from build123d import *

# Parameters (mm, degrees)
PLACA_DELANTERA_START               = -206
PLACA_DELANTERA_DEPTH               = 3
AGUJERO_PLACA_DELANTERA_1_PROFILE_R = 2
AGUJERO_PLACA_DELANTERA_2_PROFILE_R = 2
AGUJERO_PLACA_DELANTERA_3_PROFILE_R = 2
AGUJERO_PLACA_DELANTERA_4_PROFILE_R = 2
PLACA_TRASERA_START                 = -142
PLACA_TRASERA_DEPTH                 = 3
AGUJERO_PLACA_TRASERA_1_PROFILE_R   = 2
AGUJERO_PLACA_TRASERA_2_PROFILE_R   = 2
AGUJERO_PLACA_TRASERA_3_PROFILE_R   = 2
AGUJERO_PLACA_TRASERA_4_PROFILE_R   = 2
MARCO_INTERIOR_START                = -86
SK_MARCO_INTERIOR_W                 = 64
SK_MARCO_INTERIOR_H                 = 26
SK_MARCO_INTERIOR_R                 = 11
MARCO_INTERIOR_DEPTH                = 3
MARCO_EXTERIOR_START                = -143
SK_MARCO_EXTERIOR_W                 = 64
SK_MARCO_EXTERIOR_H                 = 26
SK_MARCO_EXTERIOR_R                 = 11
MARCO_EXTERIOR_DEPTH                = 3
CORTAR_EXTRUIR2_DEPTH               = 10


with BuildPart() as part:
    # Sk_Eje_cuerpo → Eje_cuerpo (revolve)
    with BuildSketch(Plane(origin=(0, 0, 0), x_dir=(1, 0, 0), z_dir=(0, 1, 0)), mode=Mode.PRIVATE) as eje_cuerpo_sk:
        Polygon((-183.5, 84), (-186, 84), (-186, 92), (-182.5, 92), (-182.5, 138), (-186, 138), (-186, 146), (-185.3, 149), (-183.3, 152), (-180, 154.5), (-176.5, 155.7), (-172.5, 156), (-172.5, 147), (-183.5, 147), (-183.5, 138.5), (-178.8, 138.5), (-178.8, 91.5), (-183.5, 91.5), align=None)
    revolve(eje_cuerpo_sk.sketch.rotate(Axis((-172.5, 0, -62.1), (0, 0, -1)), 180), axis=Axis((-172.5, 0, -62.1), (0, 0, -1)))



with BuildPart() as body_2:
    # Sk_Placa_delantera → Placa_delantera (new body)
    with BuildSketch(Plane(origin=(0, 0, 0), x_dir=(0, 0, -1), z_dir=(1, 0, 0)).offset(PLACA_DELANTERA_START)):
        Polygon((86, -12), (112, -12), (116, -22), (120, -12), (146, -12), (146, 10), (144.125, 14), (142.25, 10), (140.375, 14), (138.5, 10), (136.625, 14), (134.75, 10), (132.875, 14), (131, 10), (129.125, 14), (127.25, 10), (125.375, 14), (123.5, 10), (121.625, 14), (119.75, 10), (117.875, 14), (116, 10), (114.125, 14), (112.25, 10), (110.375, 14), (108.5, 10), (106.625, 14), (104.75, 10), (102.875, 14), (101, 10), (99.125, 14), (97.25, 10), (95.375, 14), (93.5, 10), (91.625, 14), (89.75, 10), (87.875, 14), (86, 10), align=None)
    extrude(amount=PLACA_DELANTERA_DEPTH)

    # Agujero_Placa_delantera_1: sweep along a curve in space
    with BuildLine() as agujero_placa_delantera_1_path:
        Line((-201.5, -6, -91), (-207.5, -6, -91))
    # Agujero_Placa_delantera_1 profile (on start of the path) → Agujero_Placa_delantera_1 (sweep, cut)
    with BuildSketch(Plane(origin=(-201.5, -6, -91), x_dir=(0, 0, -1), z_dir=(-1, 0, 0))):
        Circle(AGUJERO_PLACA_DELANTERA_1_PROFILE_R)
    sweep(path=agujero_placa_delantera_1_path.line, mode=Mode.SUBTRACT)

    # Agujero_Placa_delantera_2: sweep along a curve in space
    with BuildLine() as agujero_placa_delantera_2_path:
        Line((-201.5, 2, -91), (-207.5, 2, -91))
    # Agujero_Placa_delantera_2 profile (on start of the path) → Agujero_Placa_delantera_2 (sweep, cut)
    with BuildSketch(Plane(origin=(-201.5, 2, -91), x_dir=(0, 0, -1), z_dir=(-1, 0, 0))):
        Circle(AGUJERO_PLACA_DELANTERA_2_PROFILE_R)
    sweep(path=agujero_placa_delantera_2_path.line, mode=Mode.SUBTRACT)

    # Agujero_Placa_delantera_3: sweep along a curve in space
    with BuildLine() as agujero_placa_delantera_3_path:
        Line((-201.5, -6, -141), (-207.5, -6, -141))
    # Agujero_Placa_delantera_3 profile (on start of the path) → Agujero_Placa_delantera_3 (sweep, cut)
    with BuildSketch(Plane(origin=(-201.5, -6, -141), x_dir=(0, 0, -1), z_dir=(-1, 0, 0))):
        Circle(AGUJERO_PLACA_DELANTERA_3_PROFILE_R)
    sweep(path=agujero_placa_delantera_3_path.line, mode=Mode.SUBTRACT)

    # Agujero_Placa_delantera_4: sweep along a curve in space
    with BuildLine() as agujero_placa_delantera_4_path:
        Line((-201.5, 2, -141), (-207.5, 2, -141))
    # Agujero_Placa_delantera_4 profile (on start of the path) → Agujero_Placa_delantera_4 (sweep, cut)
    with BuildSketch(Plane(origin=(-201.5, 2, -141), x_dir=(0, 0, -1), z_dir=(-1, 0, 0))):
        Circle(AGUJERO_PLACA_DELANTERA_4_PROFILE_R)
    sweep(path=agujero_placa_delantera_4_path.line, mode=Mode.SUBTRACT)


with BuildPart() as body_3:
    # Sk_Placa_trasera → Placa_trasera (new body)
    with BuildSketch(Plane(origin=(0, 0, 0), x_dir=(0, 0, -1), z_dir=(1, 0, 0)).offset(PLACA_TRASERA_START)):
        Polygon((86, -12), (146, -12), (146, 10), (144.125, 14), (142.25, 10), (140.375, 14), (138.5, 10), (136.625, 14), (134.75, 10), (132.875, 14), (131, 10), (129.125, 14), (127.25, 10), (125.375, 14), (123.5, 10), (121.625, 14), (119.75, 10), (117.875, 14), (116, 10), (114.125, 14), (112.25, 10), (110.375, 14), (108.5, 10), (106.625, 14), (104.75, 10), (102.875, 14), (101, 10), (99.125, 14), (97.25, 10), (95.375, 14), (93.5, 10), (91.625, 14), (89.75, 10), (87.875, 14), (86, 10), align=None)
    extrude(amount=PLACA_TRASERA_DEPTH)

    # Agujero_Placa_trasera_1: sweep along a curve in space
    with BuildLine() as agujero_placa_trasera_1_path:
        Line((-137.5, -6, -91), (-143.5, -6, -91))
    # Agujero_Placa_trasera_1 profile (on start of the path) → Agujero_Placa_trasera_1 (sweep, cut)
    with BuildSketch(Plane(origin=(-137.5, -6, -91), x_dir=(0, 0, -1), z_dir=(-1, 0, 0))):
        Circle(AGUJERO_PLACA_TRASERA_1_PROFILE_R)
    sweep(path=agujero_placa_trasera_1_path.line, mode=Mode.SUBTRACT)

    # Agujero_Placa_trasera_2: sweep along a curve in space
    with BuildLine() as agujero_placa_trasera_2_path:
        Line((-137.5, 2, -91), (-143.5, 2, -91))
    # Agujero_Placa_trasera_2 profile (on start of the path) → Agujero_Placa_trasera_2 (sweep, cut)
    with BuildSketch(Plane(origin=(-137.5, 2, -91), x_dir=(0, 0, -1), z_dir=(-1, 0, 0))):
        Circle(AGUJERO_PLACA_TRASERA_2_PROFILE_R)
    sweep(path=agujero_placa_trasera_2_path.line, mode=Mode.SUBTRACT)

    # Agujero_Placa_trasera_3: sweep along a curve in space
    with BuildLine() as agujero_placa_trasera_3_path:
        Line((-137.5, -6, -141), (-143.5, -6, -141))
    # Agujero_Placa_trasera_3 profile (on start of the path) → Agujero_Placa_trasera_3 (sweep, cut)
    with BuildSketch(Plane(origin=(-137.5, -6, -141), x_dir=(0, 0, -1), z_dir=(-1, 0, 0))):
        Circle(AGUJERO_PLACA_TRASERA_3_PROFILE_R)
    sweep(path=agujero_placa_trasera_3_path.line, mode=Mode.SUBTRACT)

    # Agujero_Placa_trasera_4: sweep along a curve in space
    with BuildLine() as agujero_placa_trasera_4_path:
        Line((-137.5, 2, -141), (-143.5, 2, -141))
    # Agujero_Placa_trasera_4 profile (on start of the path) → Agujero_Placa_trasera_4 (sweep, cut)
    with BuildSketch(Plane(origin=(-137.5, 2, -141), x_dir=(0, 0, -1), z_dir=(-1, 0, 0))):
        Circle(AGUJERO_PLACA_TRASERA_4_PROFILE_R)
    sweep(path=agujero_placa_trasera_4_path.line, mode=Mode.SUBTRACT)


with BuildPart() as part_1:
    add(part.part)

    add(body_2.part)  # Marco_interior merges body 2

    add(body_3.part)  # Marco_interior merges body 3
    # Sk_Marco_interior → Marco_interior (add)
    with BuildSketch(Plane.XY.offset(MARCO_INTERIOR_START)):
        with Locations((-172.5, 0)):
            Rectangle(SK_MARCO_INTERIOR_W, SK_MARCO_INTERIOR_H)
        with Locations((-172.5, 0)):
            Circle(SK_MARCO_INTERIOR_R, mode=Mode.SUBTRACT)
    extrude(amount=-MARCO_INTERIOR_DEPTH)

    # Sk_Marco_exterior → Marco_exterior (add)
    with BuildSketch(Plane.XY.offset(MARCO_EXTERIOR_START)):
        with Locations((-172.5, 0)):
            Rectangle(SK_MARCO_EXTERIOR_W, SK_MARCO_EXTERIOR_H)
        with Locations((-172.5, 0)):
            Circle(SK_MARCO_EXTERIOR_R, mode=Mode.SUBTRACT)
    extrude(amount=-MARCO_EXTERIOR_DEPTH)

    # Croquis1 → Cortar-Extruir2 (cut)
    with BuildSketch(Plane(origin=(-139, 0, 0), x_dir=(0, 0, -1), z_dir=(1, 0, 0))):
        with BuildLine():
            Line((117.492022853, -1), (117.492022853, -5))
            ThreePointArc((117.492022853, -5), (118.370702509, -7.121320344), (120.492022853, -8))
            Line((120.492022853, -8), (141, -8))
            Line((141, -8), (141, 2))
            Line((141, 2), (120.492022853, 2))
            ThreePointArc((120.492022853, 2), (118.370702509, 1.121320344), (117.492022853, -1))
        make_face()
    cortar_extruir2 = extrude(amount=-CORTAR_EXTRUIR2_DEPTH, mode=Mode.SUBTRACT)

    # Simetr_a1: Cortar-Extruir2 across plane
    add(cortar_extruir2.mirror(Plane(origin=(-173, 0, 0), x_dir=(0, 0, 1), z_dir=(1, 0, 0))), mode=Mode.SUBTRACT)


solid = part_1.part
Can you work these out from the model? Positions are in its coordinate system, mm. A direction names the side the tool comes from. Coordinates: 2 decimals unless noted, no trailing zeros. Loops run counter-clockwise (first coordinate to the right, second up) from the corner with the lowest first, then second, coordinate; pieces in that order, holes last. Notation, with made-up numbers: (-38.75, -37.5) - (-21.75, -37.5) arc R31 ccw to (-21.75, -12.5) - close; hole circle Ø2 at (-22, -20.5). An arc over 180 degrees is marked (long way). Put each result on its own line as item: value. Start each with the question number.
Item 1: If we mould it in two halves opening along Y, with no side actions, what happens to faces 4 (the face through (-204.521, -6.601, -92.908)), 5 (the face through (-178.794, -0.277, -114.671)), 6 (the face through (-185.987, -0.594, -89.834)), 7 (the face through (-161, 0, -84))? For each: +Y half, -Y half, draft (parallel to the pull), parting line (faces both ways), or undercut.
Item 2: Suppose I cut it at C-C (y = 9). State how many separate pieces and enclosed holes the cut face has, and give its area (3 significant figures).
Item 3: Suppose I cut it at A-A (x = -151). Please give me the cut outline in (y, z), and give its area (3 significant figures).
Item 4: Which directions (+Z, -Z, +X, -X, +Y, -Y) give clear straight access to the entire face, cutting with the end or side of a thin tool? Please do faces 1 (the face through (-140.521, 3.46, -142.367)), 2 (the face through (-203, 0, -116)), 3 (the face through (-139, 1, -109)).
Item 5: If I drill on line 1 along X through (y, z) = (12.5, -106.5); line 2 along Z through (x, y) = (-157.5, -9.5); line 3 along Y through (x, z) = (-172.5, -87.5), over which ranges is the centre line in solid material (lowest first)?
Item 6: For pin 1 (2.5 mm diameter, centred on x = -141, z = -109.5, fed in from -Y); pin 2 (0.9 mm diameter, centred on x = -140.5, y = -2.5, fed in from +Z); pin 3 (0.5 mm diameter, centred on y = -12.5, z = -87, fed in from -X); pin 4 (6 mm diameter, centred on y = -5.5, z = -136.5, fed in from -X), each with a flat end and sliding along its axis, tell me the tip position at first contact or that it passes through.
Item 7: Suppose I cut it at B-B (y = -14.5). Please give me the cut outline in (x, z), and give its area (3 significant figures).
Here are the results:
1. face 4: undercut
1. face 5: undercut
1. face 6: parting line
1. face 7: draft
2. separate pieces: 1
2. enclosed holes: 3
2. area: 1,240 mm²
3. outline: (-13, -146) - (13, -146) - (13, -143) - (-13, -143) - close; (-13, -89) - (13, -89) - (13, -86) - (-13, -86) - close
3. area: 156 mm²
4. face 1: +X
4. face 2: +Y, -Y
4. face 3: +Z, -Z, +X, +Y, -Y
5. line 1: -206 to -203, -142 to -139
5. line 2: -146 to -143, -89 to -86
5. line 3: -13.5 to -11, 11 to 13.5
6. pin 1: y = -12
6. pin 2: z = -86
6. pin 3: x = -204.5
6. pin 4: x = -206
7. outline: (-206, -119) - (-203, -119) - (-203, -113) - (-206, -113) - close
7. area: 18.0 mm²
